Could you check a few things on this drawing? It's one solid part, dimensions in mm from its lowest x, y, z. Coordinates: 2 decimals unless noted, no trailing zeros. Loops run counter-clockwise (first coordinate to the right, second up) from the corner with the lowest first, then second, coordinate; pieces in that order, holes last. Notation, with made-up numbers: M 31,58 L 87,58 A37 cw 87,94 Z; hole C 58,5 d9. An arc over 180 degrees is marked long. Use one line per item in the form item = value. Start each with the question number.
(1) Thinking about a two-plate mould opening in Y: for the marked faces 1 and 2, which applies, +Y half, -Y half, draft (parallel to the pull), parting line (faces both ways), or undercut?
(2) Please list where these lines run through material, in increasing order: L1, parallel to X at y = 5.75, z = 69; L2, parallel to Y at x = 40.5, z = 33.5.
(3) Imagine slicing it at A-A, the plane z = 27.5. Please give me the cut outline in (x, y), and give its area (3 significant figures).
(4) Will this pin go through, and if not, where does the flat tip stop? P1, Ø0.6, axis at x = 25.5, z = 24.5, coming from the +Y side.
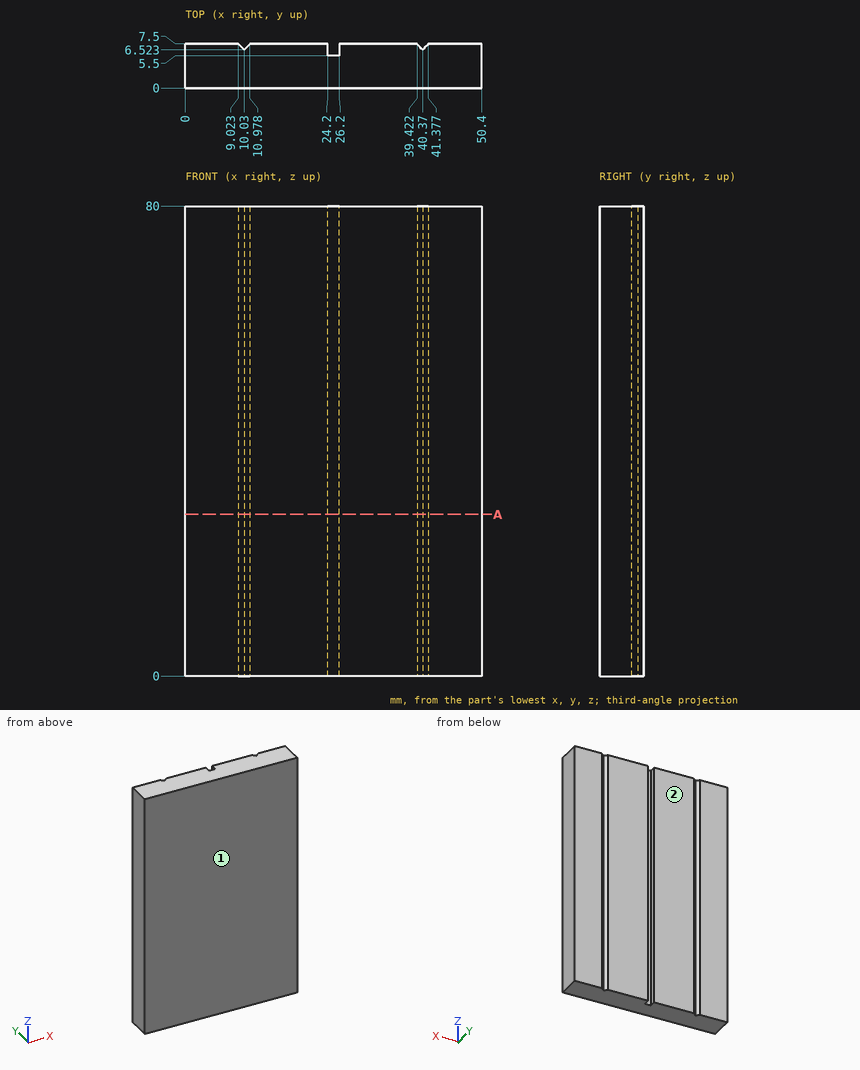
Answer:
q1.face_1 = -Y half
q1.face_2 = +Y half
q2.L1 = 0 to 24.2, 26.2 to 50.4
q2.L2 = 0 to 6.65
q3.outline = M 0,0 L 50.4,0 L 50.4,7.5 L 41.38,7.5 L 40.37,6.52 L 39.42,7.5 L 26.2,7.5 L 26.2,5.5 L 24.2,5.5 L 24.2,7.5 L 10.98,7.5 L 10.03,6.52 L 9.02,7.5 L 0,7.5 Z
q3.area = 372 mm²
q4.P1 = 5.5
